from build123d import *

# Parameters (mm, degrees)
BOSS_EXTRUDE1_DEPTH = 12
SKETCH_2_R          = 6.75
CUT_EXTRUDE1_DEPTH  = 8.5
SKETCH_4_R          = 7.5
BOSS_EXTRUDE2_DEPTH = 3
SKETCH_3_R          = 3.4
CUT_EXTRUDE2_DEPTH  = 33.74522866
FILLET1_SIZE        = 0.2


with BuildPart() as part:
    # 草图1 → Boss-Extrude1 (new body)
    with BuildSketch(Plane(origin=(0, 0, 0), x_dir=(1, 0, 0), z_dir=(0, 1, 0))):
        with BuildLine():
            Line((-5, -28), (-5, -8.660254038))
            ThreePointArc((-5, -8.660254038), (-10, 0), (-5, 8.660254038))
            Line((-5, 8.660254038), (-5, 28))
            ThreePointArc((-5, 28), (-4.414213562, 29.414213562), (-3, 30))
            Line((-3, 30), (3, 30))
            ThreePointArc((3, 30), (4.414213562, 29.414213562), (5, 28))
            Line((5, 28), (5, 8.660254038))
            ThreePointArc((5, 8.660254038), (10, 0), (5, -8.660254038))
            Line((5, -8.660254038), (5, -28))
            ThreePointArc((5, -28), (4.414213562, -29.414213562), (3, -30))
            Line((3, -30), (-3, -30))
            ThreePointArc((-3, -30), (-4.414213562, -29.414213562), (-5, -28))
        make_face()
    extrude(amount=BOSS_EXTRUDE1_DEPTH)

    # 草图2 → Cut-Extrude1 (cut)
    with BuildSketch(Plane.XZ):
        with Locations(Location((0, 0, 0), (0, 0, 270))):
            Circle(SKETCH_2_R)
    extrude(amount=-CUT_EXTRUDE1_DEPTH, mode=Mode.SUBTRACT)

    # 草图4 → Boss-Extrude2 (add)
    with BuildSketch(Plane(origin=(0, 12, 0), x_dir=(1, 0, 0), z_dir=(0, 1, 0))):
        with Locations(Location((0, 0, 0), (0, 0, 270))):
            Circle(SKETCH_4_R)
    extrude(amount=BOSS_EXTRUDE2_DEPTH)

    # 草图3 → Cut-Extrude2 (cut, through all)
    with BuildSketch(Plane.XZ.offset(-8.5)):
        with Locations(Location((0, 0, 0), (0, 0, 270))):
            Circle(SKETCH_3_R)
    extrude(amount=-CUT_EXTRUDE2_DEPTH, mode=Mode.SUBTRACT)

    # Fillet1
    fillet1_edges = [part.edges().sort_by_distance(p)[0] for p in [
        (5, 0, 18.330127019),
        (4.414213562, 0, 29.414213562),
        (4.414213562, 12, -29.414213562),
        (0, 0, 30),
        (-4.414213562, 0, 29.414213562),
        (-5, 0, 18.330127019),
        (-10, 0, 0),
        (-5, 0, -18.330127019),
        (-4.414213562, 0, -29.414213562),
        (0, 0, -30),
        (4.414213562, 0, -29.414213562),
        (5, 0, -18.330127019),
        (10, 0, 0),
        (0, 12, -30),
        (-4.414213562, 12, -29.414213562),
        (-5, 12, -18.330127019),
        (-10, 12, 0),
        (-5, 12, 18.330127019),
        (-4.414213562, 12, 29.414213562),
        (0, 0, 6.75),
        (0, 12, 30),
        (0, 15, -7.5),
        (4.414213562, 12, 29.414213562),
        (0, 15, 3.4),
        (5, 12, 18.330127019),
        (10, 12, 0),
        (5, 12, -18.330127019),
    ]]
    chamfer(fillet1_edges, length=FILLET1_SIZE)


solid = part.part
The listing builds one solid part. Answer for the finished solid, in the listing's coordinates (mm). A direction names the side the tool comes from. Coordinates: 2 decimals unless noted, no trailing zeros. Loops run counter-clockwise (first coordinate to the right, second up) from the corner with the lowest first, then second, coordinate; pieces in that order, holes last.
1) Find section A-A on z = 0. Write down the section's boundary in (x, y).
2) Determine the mould class of faces 1 (the face through (-3.32, 11.61, 0.74)), 2 (the face through (1.72, 15, -3.35)), 3 (the face through (5, 6, 18)) for opening direction X: pulls with the +X half, pulls with the -X half, needs draft (parallel to the pull), parting line crosses it, or undercut.
3) Find section C-C on x = 0. Write down the section's boundary in (y, z).
4) Find section B-B on y = 9.5. Write down the section's boundary in (x, z).
5) Flat-ended cylindrical pins translate along their axes: pin 1 Ø6 at (y, z) = (5.5, -17) entering from -X; pin 2 Ø1.5 at (y, z) = (9.5, 15.5) entering from +X; pin 3 Ø6 at (x, z) = (-3, 13) entering from +Y; pin 4 Ø10 at (x, z) = (6, -11.5) entering from -Y. Find the tip coordinate at first contact, or state that the pin passes through.
6) A tool of negligible diameter and unlimited length cuts with its end or side. For faces 4 (the face through (4.4, 5.92, -29.43)), 5 (the face through (-6.59, 4.29, 1.46)), 6 (the face through (0.33, 13.38, -7.493)), from which of +Z, -Z, +X, -X, +Y, -Y can it reach the whole face along a straight path? Write none if from no direction.
7) Find section D-D on z = -22. Write down the section's boundary in (x, y).
8) Find the intervals of material crossed by L1, parallel to X at y = 13.75, z = 0; L2, parallel to Y at x = 0.75, z = -8.5; L3, parallel to Y at x = -5, z = -4.5, in increasing order.
Values:
1. outline: (-10, 0.2) - (-9.8, 0) - (-6.95, 0) - (-6.75, 0.2) - (-6.75, 8.5) - (-3.4, 8.5) - (-3.4, 14.8) - (-3.6, 15) - (-7.3, 15) - (-7.5, 14.8) - (-7.5, 12) - (-9.8, 12) - (-10, 11.8) - close; (3.4, 8.5) - (6.75, 8.5) - (6.75, 0.2) - (6.95, 0) - (9.8, 0) - (10, 0.2) - (10, 11.8) - (9.8, 12) - (7.5, 12) - (7.5, 14.8) - (7.3, 15) - (3.6, 15) - (3.4, 14.8) - close
2. face 1: undercut
2. face 2: needs draft
2. face 3: pulls with the +X half
3. outline: (0, -29.8) - (0.2, -30) - (11.8, -30) - (12, -29.8) - (12, -7.5) - (14.8, -7.5) - (15, -7.3) - (15, -3.6) - (14.8, -3.4) - (8.5, -3.4) - (8.5, -6.75) - (0.2, -6.75) - (0, -6.95) - close; (0, 6.95) - (0.2, 6.75) - (8.5, 6.75) - (8.5, 3.4) - (14.8, 3.4) - (15, 3.6) - (15, 7.3) - (14.8, 7.5) - (12, 7.5) - (12, 29.8) - (11.8, 30) - (0.2, 30) - (0, 29.8) - close
4. outline: (-5, -28) arc R2 ccw to (-3, -30) - (3, -30) arc R2 ccw to (5, -28) - (5, -8.66) arc R10 ccw to (5, 8.66) - (5, 28) arc R2 ccw to (3, 30) - (-3, 30) arc R2 ccw to (-5, 28) - (-5, 8.66) arc R10 ccw to (-5, -8.66) - close; hole circle Ø6.8 at (0, 0)
5. pin 1: stops at x = -5
5. pin 2: stops at x = 5
5. pin 3: stops at y = 12
5. pin 4: stops at y = 0
6. face 4: -Z, +X, +Y, -Y
6. face 5: -Y
6. face 6: +Y
7. outline: (-5, 0.2) - (-4.8, 0) - (4.8, 0) - (5, 0.2) - (5, 11.8) - (4.8, 12) - (-4.8, 12) - (-5, 11.8) - close
8. L1: x = -7.5 to -3.4, 3.4 to 7.5
8. L2: y = 0 to 12
8. L3: y = 8.5 to 15
